```python
from build123d import *

# Parameters (mm, degrees)
SZKIC1_W                    = 110
SZKIC1_H                    = 14
DODANIE_WYCI_GNI_CIE1_DEPTH = 6
SZKIC2_W                    = 5.4
SZKIC2_H                    = 5.55
WYTNIJ_WYCI_GNI_CIE1_DEPTH  = 6
WYTNIJ_WYCI_GNI_CIE2_DEPTH  = 6


with BuildPart() as part:
    # Szkic1 → Dodanie-wyciągnięcie1 (new body)
    with BuildSketch(Plane(origin=(0, 0, 0), x_dir=(1, 0, 0), z_dir=(0, 1, 0))):
        with Locations((55, -89.241330813)):
            Rectangle(SZKIC1_W, SZKIC1_H)
    extrude(amount=DODANIE_WYCI_GNI_CIE1_DEPTH)

    # Szkic2 → Wytnij-wyciągnięcie1 (cut)
    with BuildSketch(Plane(origin=(0, 6, 0), x_dir=(1, 0, 0), z_dir=(0, 1, 0))):
        with Locations((2.7, -89.241330813)):
            Rectangle(SZKIC2_W, SZKIC2_H)
    extrude(amount=-WYTNIJ_WYCI_GNI_CIE1_DEPTH, mode=Mode.SUBTRACT)

    # Szkic3 → Wytnij-wyciągnięcie2 (cut)
    with BuildSketch(Plane(origin=(0, 6, 0), x_dir=(1, 0, 0), z_dir=(0, 1, 0))):
        Polygon((106.795706006, -92.016330813), (110, -92.016330813), (111.602146997, -89.241330813), (110, -86.466330813), (106.795706006, -86.466330813), (105.193559009, -89.241330813), align=None)
    extrude(amount=-WYTNIJ_WYCI_GNI_CIE2_DEPTH, mode=Mode.SUBTRACT)


solid = part.part
```
Verification items for the finished model (mm, model axes). A direction names the side the tool comes from. Give positions to 0.01 mm unless a question says otherwise; leave off trailing zeros. Order: outer loops, then holes, each group sorted by start corner. A loop starts at its lowest first (then second) coordinate and runs counter-clockwise, first axis right, second up. Notation, with made-up numbers: (-30.5, 48.25) -> (-8.5, 48.25) arc R25 ccw to (-8.5, 78.25) -> close; hole circle Ø3 at (-8, 38.25). An arc over 180 degrees is marked (long way). One line per item, written item: value.
(1) Sectioned sample at B-B on z = 87.5. Record the cut outline in (x, y).
Final values:
outline: (5.4, 0) -> (106.2, 0) -> (106.2, 6) -> (5.4, 6) -> close
(2) Gauge pin test, flat end, axial feed: pin 1 (3 mm diameter, centred on y = 3.5, z = 91, fed in from -X). Record the tip position at first contact, or that the pin passes through.
Final values:
pin 1: x = 0
(3) Tool access check on faces 5 (the face through (108, 3, 86.466)), 6 (the face through (110, 3, 94)), 7 (the face through (3, 3, 86.466)). Record the directions out of +Z, -Z, +X, -X, +Y, -Y that give a thin tool (end or side, any length) a straight path to the whole face; none if there is none.
Final values:
face 5: +X, +Y, -Y
face 6: +Z, -Z, +X, +Y, -Y
face 7: -X, +Y, -Y
(4) Draft check along Z on faces 1 (the face through (54, 3, 82.241)), 2 (the face through (106.01, 3.04, 87.83)), 3 (the face through (54, 3, 96.241)), 4 (the face through (54, 0, 89)). Enter one of: pulls with the +Z half, pulls with the -Z half, needs draft (parallel to the pull), parting line crosses it, or undercut.
Final values:
face 1: pulls with the -Z half
face 2: undercut
face 3: pulls with the +Z half
face 4: needs draft
(5) Scan lines: line 1 along X through (y, z) = (2.9, 86.5); line 2 along X through (y, z) = (2.2, 89.5). Record each from-to range of solid material in increasing order. Write a range as [from, to].
Final values:
line 1: [5.4, 106.78]
line 2: [5.4, 105.34]
(6) Sectioned sample at A-A on y = 1.6. Record the cut outline in (x, z), then the cut area to 3 significant figures.
Final values:
outline: (0, 82.24) -> (110, 82.24) -> (110, 86.47) -> (106.8, 86.47) -> (105.19, 89.24) -> (106.8, 92.02) -> (110, 92.02) -> (110, 96.24) -> (0, 96.24) -> (0, 92.02) -> (5.4, 92.02) -> (5.4, 86.47) -> (0, 86.47) -> close
area: 1,490 mm^2
